Geometry: see drawing. Coordinates: mm, zero at the bounding-box minimum. Coordinates: 2 decimals unless noted, no trailing zeros. Write each loop counter-clockwise with the first axis right and the second up, starting at its lowest first coordinate (ties: lowest second). Pieces come first, ordered by that corner, then holes.
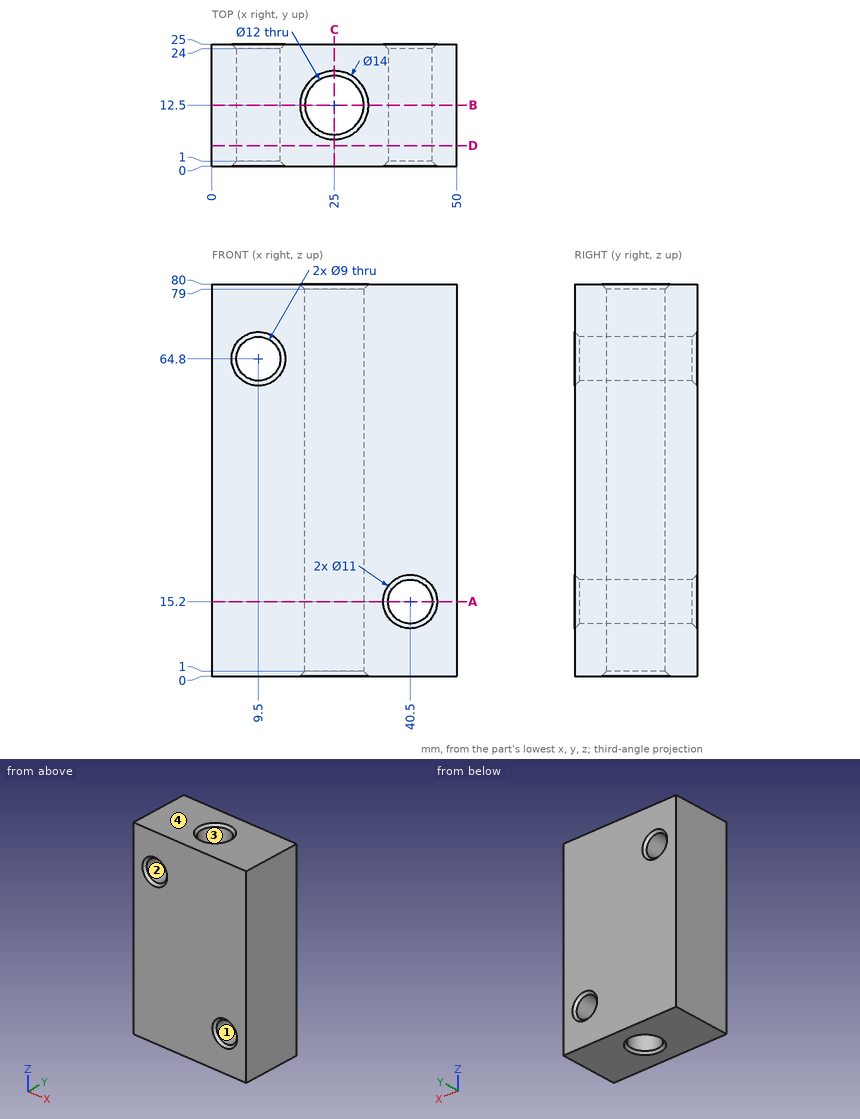
Item 1: Pull-direction query (Z, two-part tool) for the marked faces 1, 2, 3 and 4; classes: released by +Z, released by -Z, zero draft, split by the parting line, or undercut.
Derived:
face 1: undercut
face 2: undercut
face 3: zero draft
face 4: released by +Z
Item 2: Material intervals for probe 1 along X at (y, z) = (5.75, 64.8); probe 2 along X at (y, z) = (8.5, 64.8); probe 3 along X at (y, z) = (12.75, 76), sorted ascending.
Derived:
probe 1: x = 0 to 5, 14 to 50
probe 2: x = 0 to 5, 14 to 20.53, 29.47 to 50
probe 3: x = 0 to 19.01, 30.99 to 50
Item 3: Section C-C, the plane x = 25. Output: boundary loops of the cut face in (y, z).
Derived:
outline: (0, 0) - (5.5, 0) - (6.5, 1) - (6.5, 79) - (5.5, 80) - (0, 80) - close; (18.5, 1) - (19.5, 0) - (25, 0) - (25, 80) - (19.5, 80) - (18.5, 79) - close
Item 4: Section D-D, the plane y = 4.25. Output: boundary loops of the cut face in (x, z), plus the area to 3 significant figures.
Derived:
outline: (0, 0) - (50, 0) - (50, 80) - (0, 80) - close; hole circle Ø9 at (9.5, 64.8); hole circle Ø9 at (40.5, 15.2)
area: 3,870 mm2
Item 5: Section B-B, the plane y = 12.5. Output: boundary loops of the cut face in (x, z).
Derived:
outline: (0, 0) - (18, 0) - (19, 1) - (19, 79) - (18, 80) - (0, 80) - close; (31, 1) - (32, 0) - (50, 0) - (50, 80) - (32, 80) - (31, 79) - close; hole circle Ø9 at (9.5, 64.8); hole circle Ø9 at (40.5, 15.2)
Item 6: Pin query (flat end, axial travel): pin 1 (5.5 mm diameter, centred on x = 40.5, z = 15.2, fed in from -Y); pin 2 (1 mm diameter, centred on x = 24, z = 48, fed in from -Y). Return the tip coordinate at first contact, or that it passes through.
Derived:
pin 1: passes through
pin 2: stops at y = 0
Item 7: Section A-A, the plane z = 15.2. Output: boundary loops of the cut face in (x, y), plus the area to 3 significant figures.
Derived:
outline: (0, 0) - (35, 0) - (36, 1) - (36, 24) - (35, 25) - (0, 25) - close; (45, 1) - (46, 0) - (50, 0) - (50, 25) - (46, 25) - (45, 24) - close; hole circle Ø12 at (25, 12.5)
area: 910 mm2
